For this review, use the dimensioned drawing (mm, ordinates from the lowest corner) and the shaded views. Give positions to 0.01 mm unless a question says otherwise; leave off trailing zeros. Write each loop counter-clockwise with the first axis right and the second up, starting at its lowest first coordinate (ties: lowest second). Pieces come first, ordered by that corner, then holes. Notation, with made-up numbers: (-38, -34) -> (19, -34) arc R13 ccw to (19, -25) -> close; hole circle Ø7 at (-3.75, 63.25). An arc over 180 degrees is marked (long way). Return JSON: item names as keys, results as strings.
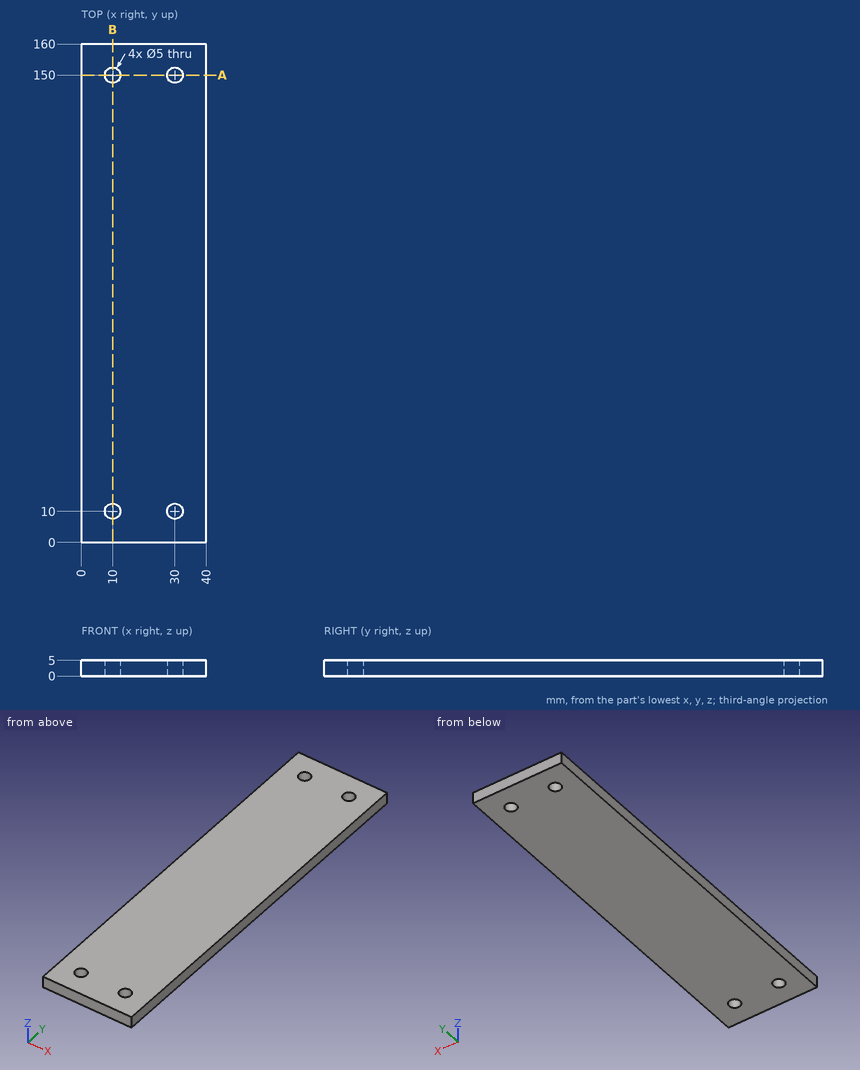
1. To check wall thickness, follow probe 1 along X at (y, z) = (150, 1.2); probe 2 along Y at (x, z) = (10, 1); probe 3 along Y at (x, z) = (31, 2.85). State the ranges of each line that lie inside material, in increasing order.
Results found:
{"probe 1": "x = 0 to 7.5, 12.5 to 27.5, 32.5 to 40", "probe 2": "y = 0 to 7.5, 12.5 to 147.5, 152.5 to 160", "probe 3": "y = 0 to 7.71, 12.29 to 147.71, 152.29 to 160"}
2. Add section A-A, the plane y = 150. State the section outline as (x, z) points.
Results found:
{"outline": "(0, 0) -> (7.5, 0) -> (7.5, 5) -> (0, 5) -> close; (12.5, 0) -> (27.5, 0) -> (27.5, 5) -> (12.5, 5) -> close; (32.5, 0) -> (40, 0) -> (40, 5) -> (32.5, 5) -> close"}
3. Add section B-B, the plane x = 10. State the section outline as (y, z) points.
Results found:
{"outline": "(0, 0) -> (7.5, 0) -> (7.5, 5) -> (0, 5) -> close; (12.5, 0) -> (147.5, 0) -> (147.5, 5) -> (12.5, 5) -> close; (152.5, 0) -> (160, 0) -> (160, 5) -> (152.5, 5) -> close"}
